```python
from build123d import *

# Parameters (mm, degrees)
F0_R     = 12.5
F1_DEPTH = 10
F2_R     = 7.55
F2_R_2   = 3.75
F3_DEPTH = 1
F4_DEPTH = 9


with BuildPart() as f1:
    # F0 (on Top) → F1 (new body)
    with BuildSketch(Plane.XY):
        with BuildLine():
            ThreePointArc((0, 17.5), (5.1256313292, 5.1256313292), (17.5, 0))
            Line((17.5, 0), (71, 0))
            ThreePointArc((71, 0), (74.5355339059, 1.4644660941), (76, 5))
            Line((76, 5), (76, 30))
            ThreePointArc((76, 30), (74.5355339059, 33.5355339059), (71, 35))
            Line((71, 35), (17.5, 35))
            ThreePointArc((17.5, 35), (5.1256313292, 29.8743686708), (0, 17.5))
        make_face()
        with Locations((17.5, 17.5)):
            Circle(F0_R, mode=Mode.SUBTRACT)
    extrude(amount=F1_DEPTH)

    # F2 (on face) → F3 (join)
    with BuildSketch(Plane.XY.offset(10)):
        with Locations((43, 17.5)):
            Circle(F2_R)
        with Locations((43, 17.5)):
            Circle(F2_R_2, mode=Mode.SUBTRACT)
        with Locations((63, 17.5)):
            Circle(F2_R)
        with Locations((63, 17.5)):
            Circle(F2_R_2, mode=Mode.SUBTRACT)
    extrude(amount=F3_DEPTH)

    # F4 (cut): faces of the model
    f4_faces = [f1.faces().sort_by_distance(p)[0] for p in [
        (43, 17.5, 10),
        (63, 17.5, 10),
    ]]
    extrude(f4_faces, amount=-F4_DEPTH, mode=Mode.SUBTRACT)


solid = f1.part
```
The listing builds one solid part. Answer for the finished solid, in the listing's coordinates (mm). A direction names the side the tool comes from. Give positions to 0.01 mm unless a question says otherwise; leave off trailing zeros. Write each loop counter-clockwise with the first axis right and the second up, starting at its lowest first coordinate (ties: lowest second). Pieces come first, ordered by that corner, then holes. Notation, with made-up numbers: M 74.25,80 L 118.25,80 A28 ccw 118.25,116 Z; hole C 52,-8 d11. An arc over 180 degrees is marked long. Write each question's results on one line, items separated by ' | '.
Q1. Section A-A, the plane z = 7.5 is taken. Write down the section's boundary in (x, y).
Output values:
outline: M 17.5,0 L 71,0 A5 ccw 76,5 L 76,30 A5 ccw 71,35 L 17.5,35 A17.5 ccw Z; hole C 17.5,17.5 d25; hole C 43,17.5 d7.5; hole C 63,17.5 d7.5
Q2. Section B-B, the plane x = 23 is taken. Write down the section's boundary in (y, z), then the cut area to 3 significant figures.
Output values:
outline: M 0,0 L 6.28,0 L 6.28,10 L 0,10 Z; M 28.72,0 L 35,0 L 35,10 L 28.72,10 Z | area: 126 mm2
Q3. Section C-C, the plane x = 63 is taken. Write down the section's boundary in (y, z).
Output values:
outline: M 0,0 L 35,0 L 35,10 L 25.05,10 L 25.05,11 L 21.25,11 L 21.25,1 L 13.75,1 L 13.75,11 L 9.95,11 L 9.95,10 L 0,10 Z
Q4. A tool of negligible diameter and unlimited length cuts with its end or side. For faces 1 (the flat face through (76, 17, 5)), 2 (the cylindrical face through (37.435, 22.603, 10.493)), from which of +Z, -Z, +X, -X, +Y, -Y can it reach the whole face along a straight path? Write none if from no direction.
Output values:
face 1: +Z, -Z, +X, +Y, -Y | face 2: +Z
Q5. Consider L1, parallel to Y at x = 17.5, z = 4.5; L2, parallel to Y at x = 63, z = 7; L3, parallel to X at y = 18, z = 8. Determine where each line is inside the solid, lowest interval first. Write a range as from..to.
Output values:
L1: 0..5, 30..35 | L2: 0..13.75, 21.25..35 | L3: 0.01..5.01, 29.99..39.28, 46.72..59.28, 66.72..76
Q6. For a pull along X with two mould halves and no side action, classify faces 3 (the cylindrical face through (14.79, 5.297, 4.93)), 4 (the cylindrical face through (40.024, 15.218, 5.93)), 5 (the cylindrical face through (75, 33, 5)), 6 (the flat face through (45, 21, 11)) as released by +X, released by -X, zero draft, split by the parting line, or undercut.
Output values:
face 3: undercut | face 4: undercut | face 5: released by +X | face 6: zero draft
Q7. Flat-ended cylindrical pins translate along their axes: P1, Ø1.5, axis at y = 22, z = 8.5, coming from the -X side; P2, Ø7, axis at x = 43, y = 17.5, coming from the +Z side; P3, Ø15, axis at x = 17.5, y = 17.5, coming from the +Z side; P4, Ø2, axis at x = 12, z = 7.5, coming from the +Y side. Find the tip coordinate at first contact, or state that the pin passes through.
Output values:
P1: x = 0.41 | P2: z = 1 | P3: through | P4: y = 34.41
Q8. Section D-D, the plane y = 3.5 is taken. Write down the section's boundary in (x, z), then the cut area to 3 significant figures.
Output values:
outline: M 7,0 L 75.77,0 L 75.77,10 L 7,10 Z | area: 688 mm2
